Autodesk Inventor part; units mm, degrees
ref_plane "Work Plane1" through (67, 0, -31.5) normal (0, 0, 1) x (1, 0, 0)
ref_plane "YZ Plane" through (0, 0, 0) normal (1, 0, 0) x (0, 1, 0)
ref_plane "XZ Plane" through (0, 0, 0) normal (0, 1, 0) x (-1, 0, 0)
sketch "Sketch1" plane through (0, 0, 0) normal (0, 0, 1) x (1, 0, 0)
  line L0 (0, 0) -> (0, -4)
  line L1 (0, -4) -> (22, -4)
  line L2 (22, -4) -> (22, -26.5)
  line L3 (22, -26.5) -> (30, -31.5)
  line L4 (30, -31.5) -> (104, -31.5)
  line L5 (104, -31.5) -> (107, -28)
  line L6 (107, -28) -> (107, 0)
  line L7 (-21.4, 0) -> (128.4, 0)
  line L8 (0, -37.8) -> (0, 6.3)
  line L9 (107, 0) -> (0, 0)
  dimension "d7" = 22.5
  dimension "d9" = 8
  dimension "d10" = 74
  dimension "d14" = 4
  dimension "d16" = 31.5
  dimension "d17" = 28
  dimension "d18" = 22
  dimension "d40" = 85
revolve "motor body" add sketch "Sketch1" angle 360 about axis through (-10, 0, 0) along (1, 0, 0)
sketch "Sketch4" plane through (0, 0, 0) normal (-1, 0, 0) x (0, 0, 1)
  circle A0 centre (0, 0) radius 4
  circle A1 centre (0, 0) radius 4
  line L0 (2.0699, 3.4228) -> (2.0699, -3.4228)
  line L1 (0, -44.1) -> (0, 44.1)
extrude "axis slot" cut sketch "Sketch4" against normal blind 25 contours A0 L0
sketch "Sketch5" plane through (22, 0, 0) normal (-1, 0, 0) x (0, 0, 1)
  circle A0 centre (15.5, 15.5) radius 1.5875
  line L0 (0, -44.1) -> (0, 44.1)
  line L1 (-44.1, 0) -> (44.1, 0)
  circle A1 centre (15.5, -15.5) radius 1.5875
  circle A2 centre (-15.5, 15.5) radius 1.5875
  circle A3 centre (-15.5, -15.5) radius 1.5875
  point P0 (0, 0)
  dimension "d22" = 3.175
  dimension "d25" = 31
  dimension "d28" = 31
  dimension "d31" = 15.5
  dimension "d32" = 15.5
extrude "mounting holes" cut sketch "Sketch5" against normal blind 4
ref_plane "Work Plane1" through (67, 0, -31.5) normal (0, 0, 1) x (1, 0, 0)
sketch "Sketch6" plane through (67, 0, -31.5) normal (0, 0, 1) x (1, 0, 0)
  line L0 (-41.25, 10) -> (-41.25, -10) construction
  line L1 (-44, 10) -> (-44, -10)
  line L2 (-38.5, -10) -> (-38.5, 10)
  arc A0 (-38.5, 10) -> (-44, 10) centre (-41.25, 10) ccw
  arc A1 (-44, -10) -> (-38.5, -10) centre (-41.25, -10) ccw
  line L3 (-45, 26.5) -> (-45, -26.5)
  line L4 (-37, 31.5) -> (-37, -31.5)
  line L5 (-92, 0) -> (62, 0)
  point P0 (-67, 0)
  point P1 (-41.25, 0)
  dimension "d35" = 20
  dimension "d36" = 5.5
  dimension "d37" = 1.5
extrude "cable hole" cut sketch "Sketch6" along normal blind 10
properties part number "motor"
Model file for the job. Use its own axes, mm. A direction names the side the tool comes from. Coordinates: 2 decimals unless noted, no trailing zeros. Loops run counter-clockwise (first coordinate to the right, second up) from the corner with the lowest first, then second, coordinate; pieces in that order, holes last. Notation, with made-up numbers: (77, -8.5) -> (87, -8.5) arc R21 ccw to (87, 19.5) -> close; hole circle Ø5 at (-36.75, 18.25). An arc over 180 degrees is marked (long way). Use one line per item in the form item = value. Start each with the question number.
(1) Cut at B-B on z = 0. Give the cut face in (x, y).
(2) Cut at A-A on y = 0. Give the cut face in (x, z) (1 decimal).
(3) Probe probe 1 along Y at (x, z) = (24.95, -15.5); probe 2 along Y at (x, z) = (24.25, -15.5); probe 3 along X at (y, z) = (-0.5, 20). List the from-to ranges inside material, lowest first. Write a range as from..to.
(4) Pull direction X, two halves, no side cores. Call faces 4 (the cylindrical face through (67.518, 4.101, -31.232)), 5 (the flat face through (28.5, 0, -26)), 6 (the flat face through (22, -6, 0)): pulls with the +X half, pulls with the -X half, needs draft (parallel to the pull), parting line crosses it, or undercut.
(5) Cut at D-D on x = 37. Give the cut face in (y, z).
(6) Cut at C-C on x = 9. Give the cut face in (y, z).
(7) Flat gauge pins, fed straight in: pin 1 (6 mm diameter, centred on x = 26.5, y = -6, fed in from -Z); pin 2 (1.5 mm diameter, centred on y = 24.5, z = -12.5, fed in from -X); pin 3 (1 mm diameter, centred on x = 61.5, z = 24, fed in from +Y). Where does each tip first touch, or does it go through?
(8) Tool access for faces 1 (the conical face through (106.81, -26.92, 8.48)), 2 (the cylindrical face through (26.634, 12.604, -24.422)), 3 (the flat face through (26, 16, -16)): list every direction of +Z, -Z, +X, -X, +Y, -Y with a clear straight run to the whole face (end or side of a thin tool).
Values:
q1.outline = (0, -4) -> (22, -4) -> (22, -26.5) -> (30, -31.5) -> (104, -31.5) -> (107, -28) -> (107, 28) -> (104, 31.5) -> (30, 31.5) -> (22, 26.5) -> (22, 4) -> (0, 4) -> close
q2.outline = (0, -4) -> (22, -4) -> (22, -26.5) -> (23, -27.1) -> (23, -21.5) -> (28.5, -21.5) -> (28.5, -30.6) -> (30, -31.5) -> (104, -31.5) -> (107, -28) -> (107, 28) -> (104, 31.5) -> (30, 31.5) -> (22, 26.5) -> (22, 4) -> (25, 4) -> (25, 2.1) -> (0, 2.1) -> close
q3.probe_1 = -23.73..-17.09, -13.91..13.91, 17.09..23.73
q3.probe_2 = -23.21..-17.09, -13.91..13.91, 17.09..23.21
q3.probe_3 = 22..107
q4.face_4 = needs draft
q4.face_5 = undercut
q4.face_6 = pulls with the -X half
q5.outline = circle Ø63 at (0, 0)
q6.outline = (-3.42, 2.07) arc R4 ccw (long way) to (3.42, 2.07) -> close
q7.pin_1 = -30.68
q7.pin_2 = 22.41
q7.pin_3 = 20.98
q8.face_1 = +X
q8.face_2 = -Z
q8.face_3 = -X
